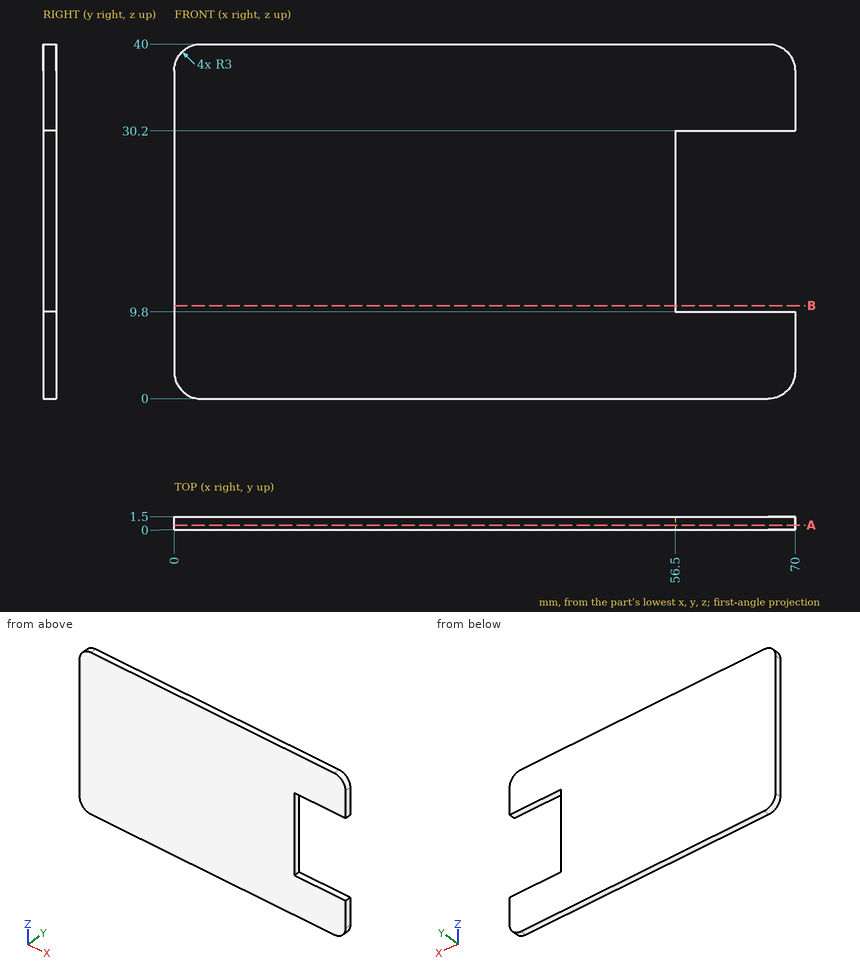
Answer from the drawing. Dimensions are ordinates in mm from the lowest x, y and z of the part. Give positions to 0.01 mm unless a question says otherwise; leave off trailing zeros. Loops run counter-clockwise (first coordinate to the right, second up) from the corner with the lowest first, then second, coordinate; pieces in that order, holes last. Notation, with made-up numbers: (-31.75, 34.5) -> (22.25, 34.5) arc R30 ccw to (22.25, 63.5) -> close; hole circle Ø2 at (82, 5.25). An arc over 180 degrees is marked (long way). One line per question, with ' | ' between items. Start each with the question number.
1) Section A-A, the plane y = 0.55 is taken. Determine the outline of the cut face in (x, z), then the cut area to 3 significant figures.
2) Straight lines are drawn through the part: L1, parallel to Z at x = 61.5, y = 0.75; L2, parallel to X at y = 1.4, z = 11. For each, find the intervals that lie inside material, in ascending order.
3) Section B-B, the plane z = 10.5 is taken. Determine the outline of the cut face in (x, y).
Resolved:
1) outline: (0, 3) arc R3 ccw to (3, 0) -> (67, 0) arc R3 ccw to (70, 3) -> (70, 9.8) -> (56.5, 9.8) -> (56.5, 30.2) -> (70, 30.2) -> (70, 37) arc R3 ccw to (67, 40) -> (3, 40) arc R3 ccw to (0, 37) -> close | area: 2,520 mm2
2) L1: 0 to 9.8, 30.2 to 40 | L2: 0 to 56.5
3) outline: (0, 0) -> (56.5, 0) -> (56.5, 1.5) -> (0, 1.5) -> close
